Source: CAD feature listing. Evaluate the final solid. Frame: model axes, mm. A direction names the side the tool comes from. Coordinates: 2 decimals unless noted, no trailing zeros. Loops run counter-clockwise (first coordinate to the right, second up) from the corner with the lowest first, then second, coordinate; pieces in that order, holes last. Notation, with made-up numbers: (-16, -14.5) -> (-10, -14.5) arc R30 cw to (-10, 18.5) -> close; hole circle Ø5 at (10, 23.5). An arc over 180 degrees is marked (long way). Answer as CSV lines item,"result".
from build123d import *

# Parameters (mm, degrees)
F1_DEPTH = 3.175


with BuildPart() as f1:
    # F0 (on Top) → F1 (new body)
    with BuildSketch(Plane.XY):
        with BuildLine():
            Line((0, 6.477), (0, 43.36577))
            ThreePointArc((0, 43.36577), (-5.051394, 45.458126), (-7.14375, 50.50952))
            Line((-7.14375, 50.50952), (-7.14375, 87.69766))
            ThreePointArc((-7.14375, 87.69766), (-13.162923, 86.99799), (-19.119664, 85.885687))
            ThreePointArc((-19.119664, 85.885687), (-23.844664, 71.210965), (-34.924976, 60.491833))
            Line((-34.924976, 60.491833), (-3.2385, 5.609247))
            ThreePointArc((-3.2385, 5.609247), (-1.676371, 6.256302), (0, 6.477))
        make_face()
        with BuildLine():
            ThreePointArc((-5.609247, 3.2385), (-4.579931, 4.579931), (-3.2385, 5.609247))
            Line((-3.2385, 5.609247), (-34.924976, 60.491833))
            ThreePointArc((-34.924976, 60.491833), (-49.748173, 56.255567), (-64.819355, 59.500958))
            ThreePointArc((-64.819355, 59.500958), (-68.761008, 54.898421), (-72.376527, 50.035499))
            Line((-72.376527, 50.035499), (-40.170653, 31.441429))
            ThreePointArc((-40.170653, 31.441429), (-36.842195, 27.103699), (-37.555859, 21.682885))
            Line((-37.555859, 21.682885), (-5.609247, 3.2385))
        make_face()
        with BuildLine():
            ThreePointArc((-6.477, 0), (-6.256302, 1.676371), (-5.609247, 3.2385))
            Line((-5.609247, 3.2385), (-37.555859, 21.682885))
            ThreePointArc((-37.555859, 21.682885), (-41.893589, 18.354428), (-47.314403, 19.068091))
            Line((-47.314403, 19.068091), (-79.520277, 37.662161))
            ThreePointArc((-79.520277, 37.662161), (-81.923931, 32.099569), (-83.939019, 26.384729))
            ThreePointArc((-83.939019, 26.384729), (-73.592836, 14.955398), (-69.849953, 0))
            Line((-69.849953, 0), (-6.477, 0))
        make_face()
        with BuildLine():
            ThreePointArc((-5.609247, -3.2385), (-6.256302, -1.676371), (-6.477, 0))
            Line((-6.477, 0), (-69.849953, 0))
            ThreePointArc((-69.849953, 0), (-73.592836, -14.955398), (-83.939019, -26.384729))
            ThreePointArc((-83.939019, -26.384729), (-81.923931, -32.099569), (-79.520277, -37.662161))
            Line((-79.520277, -37.662161), (-47.314403, -19.068091))
            ThreePointArc((-47.314403, -19.068091), (-41.893589, -18.354428), (-37.555859, -21.682885))
            Line((-37.555859, -21.682885), (-5.609247, -3.2385))
        make_face()
        with BuildLine():
            ThreePointArc((-3.2385, -5.609247), (-4.579931, -4.579931), (-5.609247, -3.2385))
            Line((-5.609247, -3.2385), (-37.555859, -21.682885))
            ThreePointArc((-37.555859, -21.682885), (-36.842195, -27.103699), (-40.170653, -31.441429))
            Line((-40.170653, -31.441429), (-72.376527, -50.035499))
            ThreePointArc((-72.376527, -50.035499), (-68.761008, -54.898421), (-64.819355, -59.500958))
            ThreePointArc((-64.819355, -59.500958), (-49.748173, -56.255567), (-34.924976, -60.491833))
            Line((-34.924976, -60.491833), (-3.2385, -5.609247))
        make_face()
        with BuildLine():
            Line((0, -43.36577), (0, -6.477))
            ThreePointArc((0, -6.477), (-1.676371, -6.256302), (-3.2385, -5.609247))
            Line((-3.2385, -5.609247), (-34.924976, -60.491833))
            ThreePointArc((-34.924976, -60.491833), (-23.844664, -71.210965), (-19.119664, -85.885687))
            ThreePointArc((-19.119664, -85.885687), (-13.162923, -86.99799), (-7.14375, -87.69766))
            Line((-7.14375, -87.69766), (-7.14375, -50.50952))
            ThreePointArc((-7.14375, -50.50952), (-5.051394, -45.458126), (0, -43.36577))
        make_face()
        with BuildLine():
            Line((34.924976, -60.491833), (3.2385, -5.609247))
            ThreePointArc((3.2385, -5.609247), (1.676371, -6.256302), (0, -6.477))
            Line((0, -6.477), (0, -43.36577))
            ThreePointArc((0, -43.36577), (5.051394, -45.458126), (7.14375, -50.50952))
            Line((7.14375, -50.50952), (7.14375, -87.69766))
            ThreePointArc((7.14375, -87.69766), (13.162923, -86.99799), (19.119664, -85.885687))
            ThreePointArc((19.119664, -85.885687), (23.844664, -71.210965), (34.924976, -60.491833))
        make_face()
        with BuildLine():
            Line((37.555859, -21.682885), (5.609247, -3.2385))
            ThreePointArc((5.609247, -3.2385), (4.579931, -4.579931), (3.2385, -5.609247))
            Line((3.2385, -5.609247), (34.924976, -60.491833))
            ThreePointArc((34.924976, -60.491833), (49.748173, -56.255567), (64.819355, -59.500958))
            ThreePointArc((64.819355, -59.500958), (68.761008, -54.898421), (72.376527, -50.035499))
            Line((72.376527, -50.035499), (40.170653, -31.441429))
            ThreePointArc((40.170653, -31.441429), (36.842195, -27.103699), (37.555859, -21.682885))
        make_face()
        with BuildLine():
            Line((69.849953, 0), (6.477, 0))
            ThreePointArc((6.477, 0), (6.256302, -1.676371), (5.609247, -3.2385))
            Line((5.609247, -3.2385), (37.555859, -21.682885))
            ThreePointArc((37.555859, -21.682885), (41.893589, -18.354428), (47.314403, -19.068091))
            Line((47.314403, -19.068091), (79.520277, -37.662161))
            ThreePointArc((79.520277, -37.662161), (81.923931, -32.099569), (83.939019, -26.384729))
            ThreePointArc((83.939019, -26.384729), (73.592836, -14.955398), (69.849953, 0))
        make_face()
        with BuildLine():
            Line((37.555859, 21.682885), (5.609247, 3.2385))
            ThreePointArc((5.609247, 3.2385), (6.256302, 1.676371), (6.477, 0))
            Line((6.477, 0), (69.849953, 0))
            ThreePointArc((69.849953, 0), (73.592836, 14.955398), (83.939019, 26.384729))
            ThreePointArc((83.939019, 26.384729), (81.923931, 32.099569), (79.520277, 37.662161))
            Line((79.520277, 37.662161), (47.314403, 19.068091))
            ThreePointArc((47.314403, 19.068091), (41.893589, 18.354428), (37.555859, 21.682885))
        make_face()
        with BuildLine():
            ThreePointArc((64.949414, 59.358962), (49.746755, 55.960011), (34.757268, 60.201354))
            Line((34.757268, 60.201354), (3.2385, 5.609247))
            ThreePointArc((3.2385, 5.609247), (4.579931, 4.579931), (5.609247, 3.2385))
            Line((5.609247, 3.2385), (37.555859, 21.682885))
            ThreePointArc((37.555859, 21.682885), (36.842195, 27.103699), (40.170653, 31.441429))
            Line((40.170653, 31.441429), (72.376527, 50.035499))
            ThreePointArc((72.376527, 50.035499), (68.821038, 54.823148), (64.949414, 59.358962))
        make_face()
        with BuildLine():
            ThreePointArc((34.757268, 60.201354), (23.589414, 71.061959), (18.931662, 85.927324))
            ThreePointArc((18.931662, 85.927324), (13.06772, 87.012341), (7.14375, 87.69766))
            Line((7.14375, 87.69766), (7.14375, 50.50952))
            ThreePointArc((7.14375, 50.50952), (5.051394, 45.458126), (0, 43.36577))
            Line((0, 43.36577), (0, 6.477))
            ThreePointArc((0, 6.477), (1.676371, 6.256302), (3.2385, 5.609247))
            Line((3.2385, 5.609247), (34.757268, 60.201354))
        make_face()
    extrude(amount=F1_DEPTH)


solid = f1.part
(1) Cut plane B-B (x = 49.5). Return the cut outline in (y, z) (3 decimals), then the cut area to 3 significant figures.
Computed values:
outline,"(-56.265, 0) -> (-36.828, 0) -> (-36.828, 3.175) -> (-56.265, 3.175) -> close; (-20.33, 0) -> (20.33, 0) -> (20.33, 3.175) -> (-20.33, 3.175) -> close; (36.828, 0) -> (55.968, 0) -> (55.968, 3.175) -> (36.828, 3.175) -> close"
area,"252 mm^2"
(2) Cut plane C-C (y = 74.5). Return the cut outline in (x, z) (3 decimals).
Computed values:
outline,"(-22.057, 0) -> (-7.144, 0) -> (-7.144, 3.175) -> (-22.057, 3.175) -> close; (7.144, 0) -> (21.755, 0) -> (21.755, 3.175) -> (7.144, 3.175) -> close"
(3) Cut plane A-A (y = 24). Return the cut outline in (x, z) (3 decimals), then the cut area to 3 significant figures.
Computed values:
outline,"(-80.814, 0) -> (-55.857, 0) -> (-55.857, 3.175) -> (-80.814, 3.175) -> close; (-36.71, 0) -> (36.71, 0) -> (36.71, 3.175) -> (-36.71, 3.175) -> close; (55.857, 0) -> (80.814, 0) -> (80.814, 3.175) -> (55.857, 3.175) -> close"
area,"392 mm^2"
(4) Draft query along X for faces 3 (the flat face through (56.05, 40.61, 1.57)), 4 (the cylindrical face through (-68.71, 54.96, 1.57)), 5 (the flat face through (63.643, 28.495, 1.565)), 6 (the cylindrical face through (81.955, 32.021, 1.565)). Return one class per face: released by +X, released by -X, zero draft, split by the parting line, or undercut.
Computed values:
face 3,"undercut"
face 4,"released by -X"
face 5,"undercut"
face 6,"released by +X"
(5) Pin query (flat end, axial travel): pin 1 Ø1 at (x, z) = (-43, 2) entering from +Y; pin 2 Ø1 at (y, z) = (-43.5, 2.5) entering from -X; pin 3 Ø1.5 at (x, z) = (62, 1) entering from -Y. Return the tip coordinate at first contact, or that it passes through.
Computed values:
pin 1,"y = 57.34"
pin 2,"x = -61.92"
pin 3,"y = -58.57"
(6) Access query for faces 1 (the flat face through (-56.5, 40.87, 1.57)), 2 (the cylindrical face through (-68.814, -54.832, 1.565)). Directions: +Z, -Z, +X, -X, +Y, -Y. A direction counts if a zero-diameter tool reaches every point of the face in a straight line with its end or side. Return the directions, or none.
Computed values:
face 1,"+Z, -Z"
face 2,"+Z, -Z, -X, -Y"
(7) Cut plane D-D (x = -31.5). Return the cut outline in (y, z) (3 decimals), then the cut area to 3 significant figures.
Computed values:
outline,"(-62.778, 0) -> (62.778, 0) -> (62.778, 3.175) -> (-62.778, 3.175) -> close"
area,"399 mm^2"
(8) Material intervals for L1, parallel to Y at x = -61.5, z = 2.4; L2, parallel to X at y = 23, z = 2.15; L3, parallel to Y at x = 48, z = 0.9, sorted ascending. Write a range as [from, to].
Computed values:
L1,"[-58.1, -43.76], [-27.26, 27.26], [43.76, 58.1]"
L2,"[-79.71, -54.12], [-36.96, 36.96], [54.12, 79.71]"
L3,"[-56.36, -35.96], [-19.46, 19.46], [35.96, 56.06]"
